Input: part model. Units: mm. Frame: model coordinates. A direction names the side the tool comes from. Coordinates: 2 decimals unless noted, no trailing zeros. Loops run counter-clockwise (first coordinate to the right, second up) from the corner with the lowest first, then second, coordinate; pieces in that order, holes last. Notation, with made-up numbers: (29.25, 4.5) -> (48.25, 4.5) arc R29 cw to (48.25, 25.5) -> close; hole circle Ø7 at (-30.5, 7). An arc over 180 degrees is marked (long way). Answer as a JSON object with one key per item and string values.
from build123d import *

# Parameters (mm, degrees)
SKETCH1_W                = 150.5
SKETCH1_H                = 30
SKETCH1_W_2              = 9.5
SKETCH1_H_2              = 9.5
BOSS_EXTRUDE1_DEPTH      = 4
SKETCH2_W                = 9.5
SKETCH2_H                = 9.5
BOSS_EXTRUDE2_DEPTH      = 12
BOSS_EXTRUDE2_DEPTH_BACK = 4
FILLET1_R                = 1
CHAMFER1_SIZE            = 0.25
CHAMFER1_SIZE2           = 8
SKETCH3_R                = 1.725
CUT_EXTRUDE1_DEPTH       = 5
SKETCH4_R                = 3
CUT_EXTRUDE2_DEPTH       = 1


with BuildPart() as part:
    # Sketch1 → Boss-Extrude1 (new body)
    with BuildSketch(Plane(origin=(0, 0, 0), x_dir=(1, 0, 0), z_dir=(0, 1, 0))):
        with Locations((75.25, 15)):
            Rectangle(SKETCH1_W, SKETCH1_H)
        with Locations((14.75, 15)):
            Rectangle(SKETCH1_W_2, SKETCH1_H_2, mode=Mode.SUBTRACT)
        with Locations((38.95, 15)):
            Rectangle(SKETCH1_W_2, SKETCH1_H_2, mode=Mode.SUBTRACT)
        with Locations((63.15, 15)):
            Rectangle(SKETCH1_W_2, SKETCH1_H_2, mode=Mode.SUBTRACT)
        with Locations((87.35, 15)):
            Rectangle(SKETCH1_W_2, SKETCH1_H_2, mode=Mode.SUBTRACT)
        with Locations((111.55, 15)):
            Rectangle(SKETCH1_W_2, SKETCH1_H_2, mode=Mode.SUBTRACT)
        with Locations((135.75, 15)):
            Rectangle(SKETCH1_W_2, SKETCH1_H_2, mode=Mode.SUBTRACT)
    extrude(amount=BOSS_EXTRUDE1_DEPTH)

    # Sketch2 → Boss-Extrude2 (add, two sides)
    with BuildSketch(Plane(origin=(0, 4, 0), x_dir=(1, 0, 0), z_dir=(0, 1, 0))) as boss_extrude2_sk:
        with Locations((14.75, 15)):
            Rectangle(SKETCH2_W, SKETCH2_H)
        with Locations((38.95, 15)):
            Rectangle(SKETCH2_W, SKETCH2_H)
        with Locations((63.15, 15)):
            Rectangle(SKETCH2_W, SKETCH2_H)
        with Locations((87.35, 15)):
            Rectangle(SKETCH2_W, SKETCH2_H)
        with Locations((111.55, 15)):
            Rectangle(SKETCH2_W, SKETCH2_H)
        with Locations((135.75, 15)):
            Rectangle(SKETCH2_W, SKETCH2_H)
    extrude(amount=BOSS_EXTRUDE2_DEPTH)
    extrude(boss_extrude2_sk.sketch, amount=-BOSS_EXTRUDE2_DEPTH_BACK)

    # Fillet1
    fillet1_edges = [part.edges().sort_by_distance(p)[0] for p in [
        (10, 16, -15),
        (14.75, 16, -10.25),
        (19.5, 16, -15),
        (14.75, 16, -19.75),
        (34.2, 16, -15),
        (38.95, 16, -10.25),
        (43.7, 16, -15),
        (38.95, 16, -19.75),
        (58.4, 16, -15),
        (63.15, 16, -10.25),
        (67.9, 16, -15),
        (63.15, 16, -19.75),
        (82.6, 16, -15),
        (87.35, 16, -10.25),
        (92.1, 16, -15),
        (87.35, 16, -19.75),
        (106.8, 16, -15),
        (111.55, 16, -10.25),
        (116.3, 16, -15),
        (111.55, 16, -19.75),
        (140.5, 16, -15),
        (135.75, 16, -19.75),
        (131, 16, -15),
        (135.75, 16, -10.25),
    ]]
    fillet(fillet1_edges, radius=FILLET1_R)

    # Chamfer1
    chamfer1_edges = [part.edges().sort_by_distance(p)[0] for p in [
        (10, 4, -15),
        (14.75, 4, -10.25),
        (19.5, 4, -15),
        (14.75, 4, -19.75),
        (58.4, 4, -15),
        (63.15, 4, -10.25),
        (67.9, 4, -15),
        (63.15, 4, -19.75),
        (34.2, 4, -15),
        (38.95, 4, -10.25),
        (43.7, 4, -15),
        (38.95, 4, -19.75),
        (82.6, 4, -15),
        (87.35, 4, -10.25),
        (92.1, 4, -15),
        (87.35, 4, -19.75),
        (106.8, 4, -15),
        (111.55, 4, -10.25),
        (116.3, 4, -15),
        (111.55, 4, -19.75),
        (140.5, 4, -15),
        (135.75, 4, -19.75),
        (131, 4, -15),
        (135.75, 4, -10.25),
    ]]
    chamfer1_side = [part.faces().sort_by_distance(p)[0] for p in [
        (75.25, 4, -15),
    ]]
    chamfer(chamfer1_edges, length=CHAMFER1_SIZE, length2=CHAMFER1_SIZE2, reference=chamfer1_side[0])

    # Sketch3 → Cut-Extrude1 (cut, through all)
    with BuildSketch(Plane(origin=(0, 4, 0), x_dir=(1, 0, 0), z_dir=(0, 1, 0))):
        with Locations((26.85, 6)):
            Circle(SKETCH3_R)
        with Locations((26.85, 24)):
            Circle(SKETCH3_R)
        with Locations((123.65, 6)):
            Circle(SKETCH3_R)
        with Locations((123.65, 24)):
            Circle(SKETCH3_R)
    extrude(amount=-CUT_EXTRUDE1_DEPTH, mode=Mode.SUBTRACT)

    # Sketch4 → Cut-Extrude2 (cut)
    with BuildSketch(Plane(origin=(0, 4, 0), x_dir=(1, 0, 0), z_dir=(0, 1, 0))):
        with Locations((26.85, 24)):
            Circle(SKETCH4_R)
        with Locations((26.85, 6)):
            Circle(SKETCH4_R)
        with Locations((123.65, 6)):
            Circle(SKETCH4_R)
        with Locations((123.65, 24)):
            Circle(SKETCH4_R)
    extrude(amount=-CUT_EXTRUDE2_DEPTH, mode=Mode.SUBTRACT)


solid = part.part
1. Line query: line 1 along X through (y, z) = (0.9, -24) (3 decimals); line 2 along Z through (x, y) = (26.85, 3.35); line 3 along X through (y, z) = (13.75, -18.25). Output: solid intervals per line, ascending.
Reply:
{"line 1": "x = 0 to 25.125, 28.575 to 121.925, 125.375 to 150.5", "line 2": "z = -30 to -27, -21 to -9, -3 to 0", "line 3": "x = 10 to 19.5, 34.2 to 43.7, 58.4 to 67.9, 82.6 to 92.1, 106.8 to 116.3, 131 to 140.5"}
2. Mould query, pull axis X, two halves, no side actions, for faces 1 (the face through (19.5, 13, -15)), 2 (the face through (116.3, 13, -15)), 3 (the face through (150.5, 2, -15)), 4 (the face through (136, 13, -19.75)). Classes: pulls with the +X half, pulls with the -X half, needs draft (parallel to the pull), parting line crosses it, or undercut.
Reply:
{"face 1": "undercut", "face 2": "undercut", "face 3": "pulls with the +X half", "face 4": "needs draft"}
3. Section query C-C (z = -6). Return loops of the section in (x, y) (3 decimals).
Reply:
{"outline": "(0, 0) -> (25.125, 0) -> (25.125, 3) -> (23.85, 3) -> (23.85, 4) -> (0, 4) -> close; (28.575, 0) -> (121.925, 0) -> (121.925, 3) -> (120.65, 3) -> (120.65, 4) -> (29.85, 4) -> (29.85, 3) -> (28.575, 3) -> close; (125.375, 0) -> (150.5, 0) -> (150.5, 4) -> (126.65, 4) -> (126.65, 3) -> (125.375, 3) -> close"}
4. Section query A-A (x = 123.65). Return loops of the section in (y, z) (3 decimals), plus the area to 3 significant figures.
Reply:
{"outline": "(0, -30) -> (4, -30) -> (4, -27) -> (3, -27) -> (3, -25.725) -> (0, -25.725) -> close; (0, -22.275) -> (3, -22.275) -> (3, -21) -> (4, -21) -> (4, -9) -> (3, -9) -> (3, -7.725) -> (0, -7.725) -> close; (0, -4.275) -> (3, -4.275) -> (3, -3) -> (4, -3) -> (4, 0) -> (0, 0) -> close", "area": "87.3 mm2"}
5. Access query for faces 5 (the face through (136, 13, -10.25)), 6 (the face through (122.28, 1.52, -4.95)). Directions: +Z, -Z, +X, -X, +Y, -Y. A direction counts if a zero-diameter tool reaches every point of the face in a straight line with its end or side. Return the directions, or none.
Reply:
{"face 5": "+Z, +X, -X, +Y", "face 6": "+Y, -Y"}
6. Pin query (flat end, axial travel): P1, Ø0.9, axis at y = 13.5, z = -15, coming from the +X side; P2, Ø2.5, axis at x = 37, y = 13, coming from the +Z side; P3, Ø1.5, axis at y = 14, z = -14.5, coming from the -X side; P4, Ø6, axis at x = 24, y = 6, coming from the -Z side. Return the tip coordinate at first contact, or that it passes through.
Reply:
{"P1": "stops at x = 140.5", "P2": "stops at z = -10.24", "P3": "stops at x = 10", "P4": "stops at z = -30"}
7. Section query B-B (y = 7.5). Return loops of the section in (x, z), plus the area to 3 significant figures.
Reply:
{"outline": "(9.86, -19.89) -> (19.64, -19.89) -> (19.64, -10.11) -> (9.86, -10.11) -> close; (34.06, -19.89) -> (43.84, -19.89) -> (43.84, -10.11) -> (34.06, -10.11) -> close; (58.26, -19.89) -> (68.04, -19.89) -> (68.04, -10.11) -> (58.26, -10.11) -> close; (82.46, -19.89) -> (92.24, -19.89) -> (92.24, -10.11) -> (82.46, -10.11) -> close; (106.66, -19.89) -> (116.44, -19.89) -> (116.44, -10.11) -> (106.66, -10.11) -> close; (130.86, -19.89) -> (140.64, -19.89) -> (140.64, -10.11) -> (130.86, -10.11) -> close", "area": "574 mm2"}
